For this review, use the dimensioned drawing (mm, ordinates from the lowest corner) and the shaded views. Coordinates: 2 decimals unless noted, no trailing zeros. Order: outer loops, then holes, each group sorted by start corner. A loop starts at its lowest first (then second) coordinate and runs counter-clockwise, first axis right, second up. Notation, with made-up numbers: M 78.25,67 L 89.25,67 A12 ccw 89.25,84 Z; hole C -34,73.5 d8. An arc over 180 degrees is marked long. Answer in a Markdown table with one row per item.
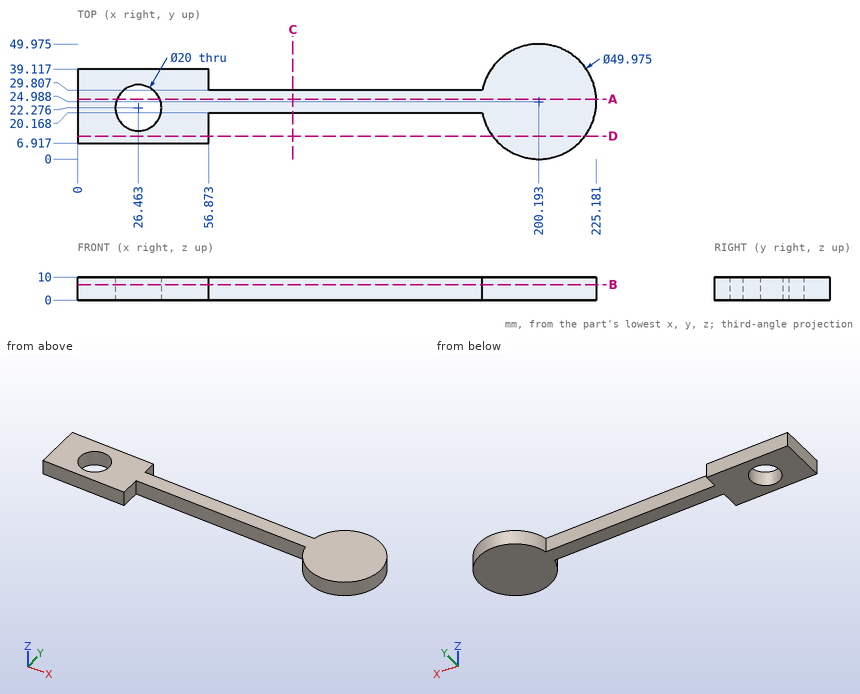
(1) Take a section at A-A (y = 26). Write out the cut boundary in (x, z) (1 decimal), then the cut area to 3 significant figures.
Report:
| item | result |
|---|---|
| outline | M 0,0 L 17.2,0 L 17.2,10 L 0,10 Z; M 35.7,0 L 225.2,0 L 225.2,10 L 35.7,10 Z |
| area | 2,070 mm^2 |
(2) Take a section at C-C (x = 93.5). Write out the cut boundary in (y, z).
Report:
| item | result |
|---|---|
| outline | M 20.17,0 L 29.81,0 L 29.81,10 L 20.17,10 Z |
(3) Take a section at B-B (z = 6.75). Write out the cut boundary in (x, y) (1 decimal).
Report:
| item | result |
|---|---|
| outline | M 0,6.9 L 56.9,6.9 L 56.9,20.2 L 175.7,20.2 A25 ccw long 175.7,29.8 L 56.9,29.8 L 56.9,39.1 L 0,39.1 Z; hole C 26.5,22.3 d20 |
(4) To check wall thickness, follow line 1 (Y direction, x = 84.5, z = 0.5); line 2 (X direction, y = 18, z = 4.75) (1 decimal); line 3 (X direction, y = 26, z = 3.5) (1 decimal). State the ranges of each line that lie inside material, in increasing order. Write a range as [from, to].
Report:
| item | result |
|---|---|
| line 1 | [20.17, 29.81] |
| line 2 | [0, 17.4], [35.5, 56.9], [176.2, 224.2] |
| line 3 | [0, 17.2], [35.7, 225.2] |
(5) Take a section at D-D (y = 10). Write out the cut boundary in (x, z).
Report:
| item | result |
|---|---|
| outline | M 0,0 L 56.87,0 L 56.87,10 L 0,10 Z; M 180.2,0 L 220.19,0 L 220.19,10 L 180.2,10 Z |
(6) Insertion check: P1, Ø4, axis at x = 29, z = 7, coming from the +Y side; P2, Ø4, axis at y = 26.5, z = 1, coming from the +X side; P3, Ø6, axis at x = 38.5, z = 3.5, coming from the -Y side. Each pin has a flat end and moves straight along its axis. Give the tip position at first contact, or say it passes through.
Report:
| item | result |
|---|---|
| P1 | y = 39.12 |
| P2 | x = 225.18 |
| P3 | y = 6.92 |
